Check sheet for the drawn part. Datum: minimum x, y, z corner. Units: mm. Round coordinates to 2 decimals unless told otherwise and drop trailing zeros. Write each loop counter-clockwise with the first axis right and the second up, starting at its lowest first coordinate (ties: lowest second). Pieces come first, ordered by that corner, then holes. Notation, with made-up numbers: M 7.25,29 L 56.25,29 A21 ccw 56.25,43 Z; hole C -6,56.25 d9. An arc over 180 degrees is marked long. Put each result on its own line as item: value.
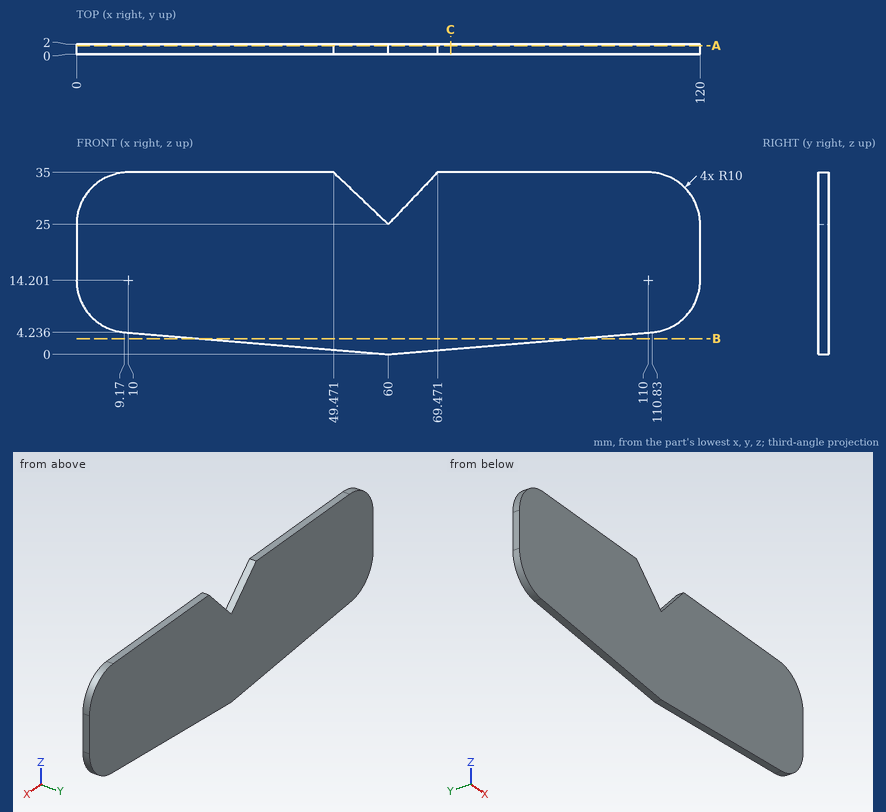
1. Cross-section at B-B (z = 3). Enter the section's corners in (x, y), then the cut area to 3 significant figures.
Computed values:
outline: M 24,0 L 96,0 L 96,2 L 24,2 Z
area: 144 mm2
2. Cross-section at C-C (x = 72). Enter the section's corners in (y, z).
Computed values:
outline: M 0,1 L 2,1 L 2,35 L 0,35 Z
3. Cross-section at A-A (y = 1.7). Enter the section's corners in (x, z) (1 decimal).
Computed values:
outline: M 0,14.2 A10 ccw 9.2,4.2 L 60,0 L 110.8,4.2 A10 ccw 120,14.2 L 120,25 A10 ccw 110,35 L 69.5,35 L 60,25 L 49.5,35 L 10,35 A10 ccw 0,25 Z
4. Scan lines: probe 1 along X at (y, z) = (1, 32); probe 2 along X at (y, z) = (0.95, 28.5) (1 decimal); probe 3 along Z at (x, y) = (65.5, 1.4) (1 decimal). Record each from-to range of solid material in increasing order.
Computed values:
probe 1: x = 2.86 to 52.63, 66.63 to 117.14
probe 2: x = 0.6 to 56.3, 63.3 to 119.4
probe 3: z = 0.5 to 30.8
